Autodesk Inventor part; units mm, degrees
ref_plane "Work Plane1" through (41.411, -174.5481, 0) normal (0, -1, 0) x (1, 0, 0)
ref_plane "YZ Plane" through (0, 0, 0) normal (1, 0, 0) x (0, 1, 0)
ref_plane "XZ Plane" through (0, 0, 0) normal (0, 1, 0) x (-1, 0, 0)
sketch "Sketch1" plane through (0, 0, 0) normal (0, 0, 1) x (1, 0, 0)
  line L0 (0, 0) -> (160, 0) construction
  line L1 (160, 0) -> (118.589, -154.5481) construction
  line L2 (0, 0) -> (41.411, -154.5481) construction
  line L3 (41.411, -154.5481) -> (118.589, -154.5481)
  circle A0 centre (235.8871, -103.156) radius 80 construction
  line L4 (160, 0) -> (256.5926, -25.8819)
  line L5 (118.589, -154.5481) -> (215.1815, -180.43)
  arc A1 (215.1815, -180.43) -> (256.5926, -25.8819) centre (235.8871, -103.156) ccw
  circle A2 centre (-75.8871, -103.156) radius 80 construction
  line L6 (0, 0) -> (-96.5926, -25.8819)
  line L7 (41.411, -154.5481) -> (-55.1815, -180.43)
  arc A3 (-96.5926, -25.8819) -> (-55.1815, -180.43) centre (-75.8871, -103.156) ccw
  arc A4 (160, 0) -> (0, 0) centre (80, -304.672) ccw
  dimension "d0" = 160
  dimension "d1" = 160
  dimension "d2" = 160
  dimension "d3" = 75
  dimension "d4" = 75
  dimension "d5" = 160
  dimension "d6" = 100
  dimension "d7" = 160
  dimension "d9" = 100
  dimension "d56" = 315
extrude "Extrusion1" add sketch "Sketch1" along normal blind 33.9
sketch "Sketch2" plane through (0, 0, 33.9) normal (0, 0, 1) x (1, 0, 0)
  line L0 (-26.5, -133) -> (186.5, -133)
  line L1 (186.5, -133) -> (186.5, -20)
  line L2 (186.5, -20) -> (-26.5, -20)
  line L3 (-26.5, -20) -> (-26.5, -133)
  line L4 (0, 0) -> (-96.5926, -25.8819)
  arc A0 (160, 0) -> (0, 0) centre (80, -304.672) ccw
  line L5 (0, 0) -> (160, 0)
  point P0 (80, -20)
  point P1 (80, 0)
  dimension "d12" = 213
  dimension "d13" = 113
  dimension "d57" = 20
extrude "Extrusion2" cut sketch "Sketch2" against normal through all contours L3 L2 L1 L0
sketch "Sketch3" plane through (0, 0, 33.9) normal (0, 0, 1) x (1, 0, 0)
  line L0 (186.5, -20) -> (186.5, -133) construction
  line L1 (186.5, -133) -> (-26.5, -133) construction
  line L2 (-26.5, -133) -> (-26.5, -20) construction
  line L3 (-26.5, -20) -> (186.5, -20) construction
  line L4 (0, 0) -> (-96.5926, -25.8819) construction
  arc A0 (-96.5926, -25.8819) -> (-55.1815, -180.43) centre (-75.8871, -103.156) ccw construction
  line L5 (-55.1815, -180.43) -> (41.411, -154.5481) construction
  line L6 (41.411, -154.5481) -> (118.589, -154.5481) construction
  line L7 (118.589, -154.5481) -> (215.1815, -180.43) construction
  arc A1 (215.1815, -180.43) -> (256.5926, -25.8819) centre (235.8871, -103.156) ccw construction
  line L8 (256.5926, -25.8819) -> (160, 0) construction
  line L9 (-48.0481, -154.5481) -> (208.0481, -154.5481) construction
  line L10 (208.0481, -154.5481) -> (208.0481, 10.328) construction
  line L11 (-48.0481, 10.328) -> (-48.0481, -154.5481) construction
  line L12 (-48.0481, 10.328) -> (-48.0481, -178.5186)
  line L13 (-55.1815, -180.43) -> (41.411, -154.5481)
  line L14 (208.0481, 10.328) -> (208.0481, -178.5186)
  line L15 (118.589, -154.5481) -> (215.1815, -180.43)
  line L16 (-48.0481, -178.5186) -> (208.0481, -178.5186)
  line L17 (-48.0481, 10.328) -> (208.0481, 10.328)
  line L18 (-157.6505, -218.8456) -> (317.6505, -218.8456)
  line L19 (317.6505, -218.8456) -> (317.6505, 50.655)
  line L20 (317.6505, 50.655) -> (-157.6505, 50.655)
  line L21 (-157.6505, 50.655) -> (-157.6505, -218.8456)
  arc A2 (160, 0) -> (0, 0) centre (80, -304.672) ccw
  point P0 (80, -154.5481)
  point P1 (80, 10.328)
  point P2 (208.0481, -84.0953)
  point P3 (317.6505, -84.0953)
  point P4 (80, 10.328)
  point P5 (80, -218.8456)
  dimension "d22" = 269.5006
  dimension "d23" = 475.3011
extrude "Extrusion3" cut sketch "Sketch3" against normal through all
sketch "Sketch5" plane through (0, 0, 33.9) normal (0, 0, 1) x (1, 0, 0)
  line L0 (118.589, -154.5481) -> (208.0481, -178.5186)
  line L1 (208.0481, -178.5186) -> (80, -178.5186)
  line L2 (80, -178.5186) -> (80, 10.328)
  line L3 (80, 10.328) -> (208.0481, 10.328)
  line L4 (208.0481, 10.328) -> (208.0481, -178.5186)
  arc A0 (160, 0) -> (0, 0) centre (80, -304.672) ccw
extrude "Extrusion4" cut sketch "Sketch5" against normal through all
sketch "Sketch6" plane through (0, 0, 0) normal (0, 1, 0) x (-1, 0, 0)
  circle A0 centre (17, 16.95) radius 2
  line L0 (26.5, 33.9) -> (26.5, 0)
  point P0 (26.5, 16.95)
  dimension "d24" = 4
  dimension "d58" = 9.5
extrude "Extrusion5" cut sketch "Sketch6" along normal through all both and the other way through all
sketch "Sketch7" plane through (0, 0, 0) normal (0, 1, 0) x (-1, 0, 0)
  circle A0 centre (17, 16.95) radius 2
  circle A1 centre (17, 16.95) radius 6.5
  dimension "d59" = 13
extrude "Extrusion6" cut sketch "Sketch7" against normal blind 10
ref_plane "Work Plane1" through (41.411, -174.5481, 0) normal (0, -1, 0) x (1, 0, 0)
sketch "Sketch8" plane through (41.411, -174.5481, 0) normal (0, -1, 0) x (1, 0, 0)
  circle A0 centre (-58.411, 16.95) radius 2
  circle A1 centre (-58.411, 16.95) radius 6.5
  point P0 (-41.411, 0)
  dimension "d32" = 13
extrude "Extrusion7" cut sketch "Sketch8" against normal blind 10
sketch "Sketch11" plane through (41.411, -154.5481, 0) normal (0, -1, 0) x (1, 0, 0)
  line L0 (0, 33.9) -> (38.589, 33.9)
  line L1 (0, 0) -> (0, 33.9)
  line L2 (0, 0) -> (38.589, 0)
  line L3 (38.589, 0) -> (38.589, 33.9)
  circle A0 centre (19.2945, 16.95) radius 2.5
  circle A1 centre (19.2945, 16.95) radius 6.5
  point P0 (-41.411, 0)
  point P1 (0, 16.95)
  point P2 (19.2945, 33.9)
  dimension "d73" = 5
  dimension "d74" = 13
extrude "Extrusion10" cut sketch "Sketch11" against normal blind 10 contours A1
sketch "Sketch12" plane through (-48.0481, -178.5186, 33.9) normal (-1, 0, 0) x (0, 0, 1)
  line L0 (-33.9, 0) -> (-33.9, 165.6442)
  line L1 (0, 0) -> (-33.9, 0)
  line L2 (0, 165.6442) -> (0, 0)
  line L3 (-33.9, 165.6442) -> (0, 165.6442)
  line L4 (-5, 5) -> (-28.9, 5)
  line L5 (-28.9, 5) -> (-28.9, 160.6442)
  line L6 (-28.9, 160.6442) -> (-5, 160.6442)
  line L7 (-5, 160.6442) -> (-5, 5)
  point P0 (-33.9, 178.5186)
  dimension "d43" = 5
extrude "Extrusion11" cut sketch "Sketch12" against normal blind 15 contours L4 L5 L6 L7
sketch "Sketch13" plane through (0, 0, 33.9) normal (0, 0, 1) x (1, 0, 0)
  circle A0 centre (-40.0481, -95.6966) radius 2.5
  line L0 (-48.0481, -12.8745) -> (-48.0481, -178.5186)
  point P0 (0, 0)
  point P1 (-48.0481, -95.6966)
  dimension "d46" = 5
  dimension "d47" = 8
extrude "Extrusion12" cut sketch "Sketch13" against normal through all
sketch "Sketch14" plane through (0, 0, 33.9) normal (0, 0, 1) x (1, 0, 0)
  circle A0 centre (-40.0481, -95.6966) radius 2.5
  circle A1 centre (-40.0481, -95.6966) radius 6.5
  point P0 (0, 0)
  dimension "d50" = 13
extrude "Extrusion13" cut sketch "Sketch14" against normal blind 4
sketch "Sketch15" plane through (0, 0, 0) normal (0, 0, -1) x (-1, 0, 0)
  circle A0 centre (40.0481, -95.6966) radius 2.5
  circle A1 centre (40.0481, -95.6966) radius 2.5
  circle A2 centre (40.0481, -95.6966) radius 6.5
  point P0 (0, 0)
  dimension "d53" = 13
extrude "Extrusion14" cut sketch "Sketch15" against normal blind 4
sketch "Sketch16" plane through (0, 0, 33.9) normal (0, 0, 1) x (1, 0, 0)
  line L0 (80, -20) -> (80, 10.328) construction
  circle A0 centre (80, -4.836) radius 8.25 construction
  circle A1 centre (80, -4.836) radius 15.164 construction
  arc A2 (80, -20) -> (80, 10.328) centre (80, -4.836) ccw
  arc A3 (80, -13.086) -> (80, 3.414) centre (80, -4.836) ccw
  arc A4 (80, 10.328) -> (0, 0) centre (80, -304.672) ccw
  line L1 (80, 10.328) -> (80, 3.414)
  line L2 (80, -13.086) -> (80, -20)
  dimension "d62" = 16.5
extrude "Extrusion15" add sketch "Sketch16" against normal blind 33.9
sketch "Sketch17" plane through (0, 0, 33.9) normal (0, 0, 1) x (1, 0, 0)
  arc A0 (80, -13.086) -> (80, 3.414) centre (80, -4.836) ccw construction
  circle A1 centre (80, -4.836) radius 8.25
  point P0 (0, 0)
extrude "Extrusion16" cut sketch "Sketch17" against normal through all
sketch "Sketch19" plane through (0, 0, 33.9) normal (0, 0, 1) x (1, 0, 0)
  circle A0 centre (80, -4.836) radius 8.25
  arc A1 (80, -20) -> (80, 10.328) centre (80, -4.836) ccw
  circle A2 centre (80, -4.836) radius 15.164 construction
  circle A3 centre (80, -4.836) radius 16.164
  point P0 (0, 0)
  dimension "d72" = 1
extrude "Extrusion18" cut sketch "Sketch19" against normal blind 16.95
sketch "Sketch20" plane through (60.7055, -154.5481, 16.95) normal (0, -1, 0) x (1, 0, 0)
  circle A0 centre (0, 0) radius 2.5
  point P0 (-60.7055, -16.95)
extrude "Extrusion19" cut sketch "Sketch20" against normal blind 50
properties part number "Riser Base" material "ABS Plastic"
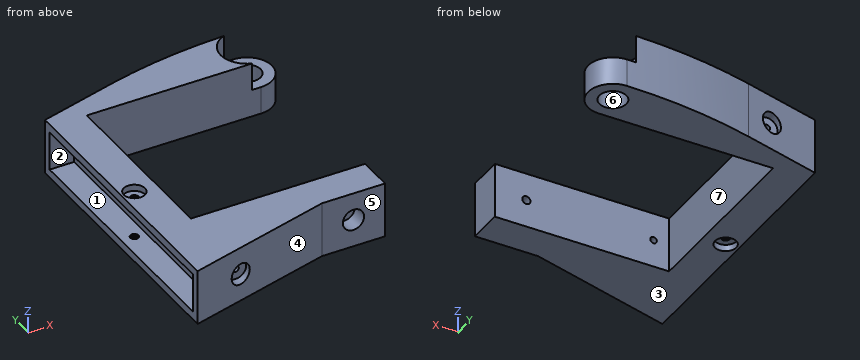
Here's how the part is built. I have some questions about the finished solid (model axes, mm). Face numbers are marked on the shaded views. A direction names the side the tool comes from. Give positions to 0.01 mm unless a question says otherwise; leave off trailing zeros. Order: outer loops, then holes, each group sorted by start corner. A loop starts at its lowest first (then second) coordinate and runs counter-clockwise, first axis right, second up. Notation, with made-up numbers: (71, 84.25) - (95, 84.25) arc R27 ccw to (95, 102.25) - close; hole circle Ø6 at (11, 35.25). An arc over 180 degrees is marked (long way). Answer as a JSON object with one key per item and string values. Group by question number.
Item 1: If we mould it in two halves opening along Z, with no side actions, what happens to the marked faces 1, 2, 3 and 4? For each: pulls with the +Z half, pulls with the -Z half, needs draft (parallel to the pull), parting line crosses it, or undercut.
Item 2: For P1, Ø16.5, axis at x = -42, z = 13.5, coming from the -Y side; P2, Ø4, axis at x = 59.5, z = 16, coming from the -Y side; P3, Ø1.5, axis at y = -86, z = 25.5, coming from the +X side, each with a flat end and sliding along its axis, tell me the tip position at first contact or that it passes through.
Item 3: Please list where these lines run through material, in increasing order: probe 1 along Z at (x, y) = (-17, -143); probe 2 along Y at (x, z) = (66.5, 19.5); probe 3 along Y at (x, z) = (0, 8).
Item 4: Which directions (+Z, -Z, +X, -X, +Y, -Y) give clear straight access to the entire face, cutting with the end or side of a thin tool? Please do the marked faces 5, 6 and 7.
Item 5: If we section it at B-B on y = -130: Please give me the cut outline in (x, z).
Item 6: If we section it at A-A on x = -17: Please give me the cut outline in (y, z).
Result set:
{
 "1": {"face 1": "undercut", "face 2": "undercut", "face 3": "pulls with the -Z half", "face 4": "needs draft"},
 "2": {"P1": "y = -178.52", "P2": "y = -144.55", "P3": "x = -26.5"},
 "3": {"probe 1": "0 to 14.95, 18.95 to 33.9", "probe 2": "-144.55 to -133, -20 to -13.73, 4.05 to 10.04", "probe 3": "-165.64 to -133, -20 to 0"},
 "4": {"face 5": "+Z, -Z, +X, -Y", "face 6": "+Z, -Z", "face 7": "+Z, -Z, +X"},
 "5": {"outline": "(-48.05, 0) - (-26.5, 0) - (-26.5, 33.9) - (-48.05, 33.9) - (-48.05, 28.9) - (-33.05, 28.9) - (-33.05, 5) - (-48.05, 5) - close"},
 "6": {"outline": "(-170.2, 0) - (-133, 0) - (-133, 14.95) - (-164.55, 14.95) - (-164.55, 10.45) - (-170.2, 10.45) - close; (-170.2, 23.45) - (-164.55, 23.45) - (-164.55, 18.95) - (-133, 18.95) - (-133, 33.9) - (-170.2, 33.9) - close; (-20, 0) - (-4.56, 0) - (-4.56, 10.45) - (-10, 10.45) - (-10, 14.95) - (-20, 14.95) - close; (-20, 18.95) - (-10, 18.95) - (-10, 23.45) - (-4.56, 23.45) - (-4.56, 33.9) - (-20, 33.9) - close"}
}
